The drawing under review shows one solid part. Ordinate dimensions are in mm from its lowest x, y, z. Give positions to 0.01 mm unless a question says otherwise; leave off trailing zeros. Loops run counter-clockwise (first coordinate to the right, second up) from the corner with the lowest first, then second, coordinate; pieces in that order, holes last. Notation, with made-up numbers: (-15.5, 31) - (38.5, 31) arc R20 ccw to (38.5, 51) - close; hole circle Ø2 at (17, 42). An arc over 180 degrees is marked (long way). Answer as CSV lines item,"result".
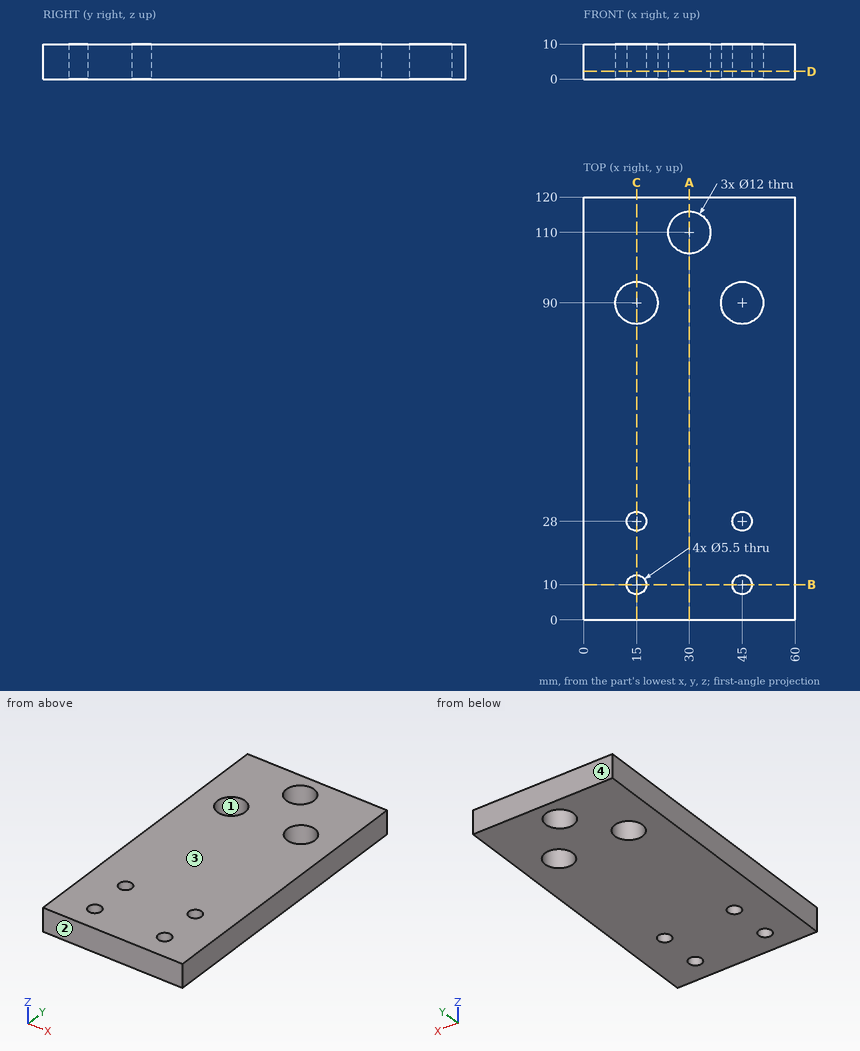
1) Consider section C-C on x = 15. Write out the cut boundary in (y, z).
From the geometry:
outline,"(0, 0) - (7.25, 0) - (7.25, 10) - (0, 10) - close; (12.75, 0) - (25.25, 0) - (25.25, 10) - (12.75, 10) - close; (30.75, 0) - (84, 0) - (84, 10) - (30.75, 10) - close; (96, 0) - (120, 0) - (120, 10) - (96, 10) - close"
2) Draft analysis for pull direction Y (two halves, no side actions). For the marked faces 1, 2, 3 and 4, state which applies: pulls with the +Y half, pulls with the -Y half, needs draft (parallel to the pull), parting line crosses it, or undercut.
From the geometry:
face 1,"undercut"
face 2,"pulls with the -Y half"
face 3,"needs draft"
face 4,"pulls with the +Y half"
3) Consider section D-D on z = 2.25. Write out the cut boundary in (x, y), and give its area (3 significant figures).
From the geometry:
outline,"(0, 0) - (60, 0) - (60, 120) - (0, 120) - close; hole circle Ø12 at (15, 90); hole circle Ø5.5 at (15, 10); hole circle Ø5.5 at (15, 28); hole circle Ø12 at (30, 110); hole circle Ø12 at (45, 90); hole circle Ø5.5 at (45, 10); hole circle Ø5.5 at (45, 28)"
area,"6,770 mm^2"
4) Consider section A-A on x = 30. Write out the cut boundary in (y, z), and give its area (3 significant figures).
From the geometry:
outline,"(0, 0) - (104, 0) - (104, 10) - (0, 10) - close; (116, 0) - (120, 0) - (120, 10) - (116, 10) - close"
area,"1,080 mm^2"
5) Consider section B-B on y = 10. Write out the cut boundary in (x, z).
From the geometry:
outline,"(0, 0) - (12.25, 0) - (12.25, 10) - (0, 10) - close; (17.75, 0) - (42.25, 0) - (42.25, 10) - (17.75, 10) - close; (47.75, 0) - (60, 0) - (60, 10) - (47.75, 10) - close"
6) Wall thickness on line 1 (Y direction, x = 45, z = 6.5); line 2 (X direction, y = 9.5, z = 4.5); line 3 (Y direction, x = 46, z = 6.5): over which ranges is each line inside the solid? List them lowest first. Write a range as from..to.
From the geometry:
line 1,"y = 0..7.25, 12.75..25.25, 30.75..84, 96..120"
line 2,"x = 0..12.3, 17.7..42.3, 47.7..60"
line 3,"y = 0..7.44, 12.56..25.44, 30.56..84.08, 95.92..120"
